```python
from build123d import *

# Parameters (mm, degrees)
SKETCH2_R             = 50
SKETCH2_R_2           = 40
BOSS_EXTRUDE1_DEPTH   = 10
SKETCH2_W             = 25
SKETCH2_H             = 5
BOSS_EXTRUDE1_2_DEPTH = 10
SKETCH3_W             = 25
SKETCH3_H             = 20
BOSS_EXTRUDE2_DEPTH   = 21.587708
SKETCH4_W             = 25
SKETCH4_H             = 10
BOSS_EXTRUDE3_DEPTH   = 30
CUT_EXTRUDE1_REACH    = 12
SKETCH5_R             = 10
FILLET1_R             = 10
FILLET2_R             = 10
FILLET3_R             = 5


with BuildPart() as part:
    # Sketch2 → Boss-Extrude1 (new body, symmetric)
    with BuildSketch(Plane.XY):
        with Locations((-261.777043848, -270)):
            Circle(SKETCH2_R)
        with Locations((-261.777043848, -270)):
            Circle(SKETCH2_R_2, mode=Mode.SUBTRACT)
    extrude(amount=BOSS_EXTRUDE1_DEPTH, both=True)



with BuildPart() as body_2:
    # Sketch2 → Boss-Extrude1 2 (new body, symmetric)
    with BuildSketch(Plane.XY):
        with Locations((-261.777043848, -197.5)):
            Rectangle(SKETCH2_W, SKETCH2_H)
    extrude(amount=BOSS_EXTRUDE1_2_DEPTH, both=True)


with BuildPart() as part_1:
    add(part.part)

    add(body_2.part)  # Boss-Extrude2 merges body 2
    # Sketch3 → Boss-Extrude2 (add)
    with BuildSketch(Plane.XZ.offset(200)):
        with Locations((-261.777043848, 0)):
            Rectangle(SKETCH3_W, SKETCH3_H)
    extrude(amount=BOSS_EXTRUDE2_DEPTH)

    # Sketch4 → Boss-Extrude3 (add)
    with BuildSketch(Plane.XY.offset(10)):
        with Locations((-261.777043848, -200)):
            Rectangle(SKETCH4_W, SKETCH4_H)
    extrude(amount=BOSS_EXTRUDE3_DEPTH)

    # Sketch5 → Cut-Extrude1 (cut, up to next)
    with BuildSketch(Plane.XZ.offset(205), mode=Mode.PRIVATE) as cut_extrude1_sk1:
        with Locations((-261.777043848, 25)):
            Circle(SKETCH5_R)
    cut_extrude1_tool1 = extrude(cut_extrude1_sk1.sketch, amount=-CUT_EXTRUDE1_REACH, mode=Mode.PRIVATE) & part_1.part
    add(cut_extrude1_tool1.solids().sort_by_distance((-261.777044, -205, 25))[0], mode=Mode.SUBTRACT)

    # Fillet1
    fillet1_edges = [part_1.edges().sort_by_distance(p)[0] for p in [
        (-274.277043848, -200, 40),
        (-249.277043848, -200, 40),
    ]]
    fillet(fillet1_edges, radius=FILLET1_R)

    # Fillet2
    fillet2_edges = [part_1.edges().sort_by_distance(p)[0] for p in [
        (-261.777043848, -195, -10),
    ]]
    fillet(fillet2_edges, radius=FILLET2_R)

    # Fillet3
    fillet3_edges = [part_1.edges().sort_by_distance(p)[0] for p in [
        (-261.777043848, -320, 10),
        (-261.777043848, -320, -10),
    ]]
    fillet(fillet3_edges, radius=FILLET3_R)


solid = part_1.part
```
Source: CAD feature listing. Evaluate the final solid. Frame: model axes, mm. A direction names the side the tool comes from. Coordinates: 2 decimals unless noted, no trailing zeros. Loops run counter-clockwise (first coordinate to the right, second up) from the corner with the lowest first, then second, coordinate; pieces in that order, holes last. Notation, with made-up numbers: M -34.75,54 L 17.25,54 A17 ccw 17.25,60 Z; hole C -10.5,30.25 d3. An arc over 180 degrees is marked long. Put each result on its own line as item: value. Start each with the question number.
1) Cut plane A-A on z = 25. Return the cut outline in (x, y).
2) Cut plane D-D on z = 36.5. Return the cut outline in (x, y).
3) Contact query for flat-ended pins moving along their axis: pin 1 Ø12 at (y, z) = (-272, 15.5) entering from +X; pin 2 Ø12.5 at (x, z) = (-256, 24.5) entering from -Y; pin 3 Ø9.5 at (y, z) = (-212.5, 3) entering from -X. Output: stop coordinate, or through.
4) Ray query, L1, parallel to X at y = -211, z = -6; L2, parallel to Y at x = -247.5, z = -5.5; L3, parallel to Z at x = -230, y = -244.5. Return the intervals inside material, ascending. Write a range as from..to.
5) Pull-direction query (Y, two-part tool) for faces 1 (the face through (-293.52, -294.34, -0.14)), 2 (the face through (-252.284, -199.93, 37.148)), 3 (the face through (-263.8, -319.96, 0.07)); classes: pulls with the +Y half, pulls with the -Y half, needs draft (parallel to the pull), parting line crosses it, or undercut.
6) Reachability of faces 4 (the face through (-265, -195, 15)), 5 (the face through (-272, -231, 10)) from +Z, -Z, +X, -X, +Y, -Y: full face, straight path, thin tool, end or side. Return the list, or none.
7) Cut plane B-B on y = -270. Return the cut outline in (x, z).
8) Cut plane C-C on x = -257.5. Give the number of separate pieces and of enclosed holes in the cut face, then the cut area to 3 significant figures.
The answers:
1. outline: M -274.28,-205 L -271.78,-205 L -271.78,-195 L -274.28,-195 Z; M -251.78,-205 L -249.28,-205 L -249.28,-195 L -251.78,-195 Z
2. outline: M -271.88,-205 L -251.68,-205 L -251.68,-195 L -271.88,-195 Z
3. pin 1: stops at x = -214.64
3. pin 2: stops at y = -205
3. pin 3: stops at x = -274.28
4. L1: x = -274.28..-249.28
4. L2: y = -317.89..-307.37, -232.63..-222.11
4. L3: z = -10..10
5. face 1: undercut
5. face 2: needs draft
5. face 3: parting line crosses it
6. face 4: +Z, -Z, +X, -X, +Y
6. face 5: +Z, +X, -X, -Y
7. outline: M -311.78,-5 A5 ccw -306.78,-10 L -301.78,-10 L -301.78,10 L -306.78,10 A5 ccw -311.78,5 Z; M -221.78,-10 L -216.78,-10 A5 ccw -211.78,-5 L -211.78,5 A5 ccw -216.78,10 L -221.78,10 Z
8. separate pieces: 3
8. enclosed holes: 0
8. area: 991 mm²
